Autodesk Inventor part; units mm, degrees
ref_plane "YZ Plane" through (0, 0, 0) normal (1, 0, 0) x (0, 1, 0)
ref_plane "XZ Plane" through (0, 0, 0) normal (0, 1, 0) x (-1, 0, 0)
ref_plane "XY Plane" through (0, 0, 0) normal (0, 0, 1) x (1, 0, 0)
sketch "Sketch1" plane through (0, 0, 0) normal (0, 1, 0) x (-1, 0, 0)
  line L0 (101.6, -101.6) -> (-101.6, -101.6)
  line L1 (-101.6, -101.6) -> (-101.6, 101.6)
  line L2 (-101.6, 101.6) -> (101.6, 101.6)
  line L3 (101.6, 101.6) -> (101.6, -101.6)
  line L4 (96.6, -96.6) -> (-96.6, -96.6)
  line L5 (-96.6, -96.6) -> (-96.6, 96.6)
  line L6 (-96.6, 96.6) -> (96.6, 96.6)
  line L7 (96.6, 96.6) -> (96.6, -96.6)
  line L8 (101.6, 101.6) -> (-40.4, 101.6)
  circle A0 centre (0, 0) radius 88.9
  circle A1 centre (0, 0) radius 109.3376
  line L9 (-40.4, 101.6) -> (-101.6, 40.4)
  line L10 (-45.4, 101.6) -> (-101.6, 45.4)
  line L11 (96.6, 96.6) -> (96.6, 101.6)
  line L12 (-45.4, 101.6) -> (-35.4, 101.6)
  line L13 (-35.4, 101.6) -> (-35.4, 96.6)
  line L14 (-35.4, 96.6) -> (-45.4, 96.6)
  line L15 (-45.4, 96.6) -> (-45.4, 101.6)
  circle A2 centre (0, 0) radius 111.3376
  point P0 (96.6, 51.2168)
  point P1 (101.6, 40.4)
  point P2 (101.6, -40.4)
  point P3 (96.6, -51.2168)
  point P4 (-96.6, 45.4)
  point P5 (-45.4, 96.6)
  dimension "d0" = 203.2
  dimension "d1" = 203.2
  dimension "d2" = 101.6
  dimension "d3" = 101.6
  dimension "d4" = 5
  dimension "d5" = 5
  dimension "d6" = 5
  dimension "d7" = 5
  dimension "d10" = 142
  dimension "d12" = 61.2
  dimension "d14" = 177.8
  dimension "d15" = 5
  dimension "d16" = 5
  dimension "d17" = 10
  dimension "d34" = 2
extrude "Extrusion1" add sketch "Sketch1" along normal blind 3 contours A2 L7 L4 | L4 A1 L7 A2 | L4 A1 L5 L9 L6 L7 | A2 L5 A1 L4 | L4 L5 A2 | A1 L6 A2 L7 | A2 L6 L7
sketch "Sketch5" plane through (0, 3, 0) normal (0, 1, 0) x (1, 0, 0)
  line L0 (-96.6, -96.6) -> (45.4, -96.6)
  circle A0 centre (0, 0) radius 88.9
  line L1 (96.6, -45.4) -> (96.6, 96.6)
  line L2 (96.6, 0) -> (89.1, 0)
  line L3 (89.1, 0) -> (89.1, 10)
  line L4 (89.1, 10) -> (96.6, 10)
  line L5 (96.6, 10) -> (96.6, 0)
  line L6 (89.1, 0) -> (96.6, 0)
  line L7 (96.6, 0) -> (96.6, -10)
  line L8 (96.6, -10) -> (89.1, -10)
  line L9 (89.1, -10) -> (89.1, 0)
  line L10 (0, 0) -> (96.6, 0)
  point P0 (10, -96.6)
  dimension "d52" = 7.5
  dimension "d53" = 7.5
  dimension "d54" = 10
  dimension "d55" = 10
extrude "Extrusion4" add sketch "Sketch5" along normal blind 15 contours L3 L4 L1 L2 | L2 L1 L8 L9
sketch "Sketch7" plane through (89.1, 3, 10) normal (0, 0, 1) x (1, 0, 0)
  line L0 (2, 10) -> (5.5, 10)
  line L1 (5.5, 10) -> (5.5, 3)
  line L2 (5.5, 3) -> (2, 3)
  line L3 (2, 3) -> (2, 10)
  line L4 (7.5, 0) -> (7.5, 15)
  line L5 (0, 0) -> (0, 15)
  line L6 (0, 15) -> (7.5, 15)
  point P0 (-89.1, -3)
  dimension "d56" = 3.5
  dimension "d57" = 2
  dimension "d58" = 2
  dimension "d59" = 5
  dimension "d60" = 7
extrude "Extrusion6" cut sketch "Sketch7" against normal through all
fillet "Fillet7" radius 3.175 2 edges at (96.6, 18, 0) (89.1, 18, 0)
sketch "Sketch8" plane through (0, 3, 0) normal (0, 1, 0) x (1, 0, 0)
  arc A0 (-101.6, -98.425) -> (-98.425, -101.6) centre (-98.425, -98.425) ccw
  line L0 (44.0849, 101.6) -> (-98.425, 101.6)
  line L1 (-101.6, 98.425) -> (-101.6, -98.425)
  line L2 (-101.6, -46.1) -> (-101.6, -76.6)
  line L3 (-96.6, -96.6) -> (-96.6, 96.6)
  line L4 (-96.6, -46.1) -> (-96.6, -76.6)
  line L5 (-101.6, -76.6) -> (-96.6, -76.6)
  line L6 (-101.6, -46.1) -> (-96.6, -46.1)
  line L7 (-98.425, -101.6) -> (101.6, -101.6)
  line L8 (0, 0) -> (-101.6, 0)
  line L9 (-101.6, 46.1) -> (-101.6, 76.6)
  line L10 (-96.6, 46.1) -> (-96.6, 76.6)
  line L11 (-101.6, 76.6) -> (-96.6, 76.6)
  line L12 (-101.6, 46.1) -> (-96.6, 46.1)
  line L13 (-96.6, -76.6) -> (-90.1, -76.6)
  line L14 (-90.1, -76.6) -> (-90.1, -46.1)
  line L15 (-90.1, -46.1) -> (-96.6, -46.1)
  line L16 (-96.6, -46.1) -> (-96.6, -76.6)
  arc A1 (-98.425, 101.6) -> (-101.6, 98.425) centre (-98.425, 98.425) ccw
  line L17 (-101.6, 46.1) -> (-101.6, 76.6)
  line L18 (-96.6, 46.1) -> (-96.6, 76.6)
  line L19 (-101.6, 76.6) -> (-96.6, 76.6)
  line L20 (-101.6, 46.1) -> (-96.6, 46.1)
  line L21 (-96.6, 76.6) -> (-90.1, 76.6)
  line L22 (-90.1, 76.6) -> (-90.1, 46.1)
  line L23 (-90.1, 46.1) -> (-96.6, 46.1)
  line L24 (-96.6, 46.1) -> (-96.6, 76.6)
  point P0 (-98.425, 98.425)
  point P1 (46.1, 101.6)
  point P2 (46.1, 96.6)
  point P3 (76.6, 96.6)
  point P4 (76.6, 101.6)
  point P5 (-46.1, 96.6)
  dimension "d64" = 30.5
  dimension "d65" = 25
  dimension "d66" = 6.5
extrude "Extrusion7" cut sketch "Sketch8" against normal through all contours L21 L22 L23 L3 | L15 L14 L13 L3
sketch "Sketch10" plane through (0, 0, 0) normal (0, -1, 0) x (1, 0, 0)
  line L0 (-90, -90) -> (-90, 90)
  line L1 (-90, 90) -> (90, 90)
  line L2 (90, 90) -> (90, -90)
  line L3 (90, -90) -> (-90, -90)
  circle A0 centre (-90, -90) radius 1
  circle A1 centre (-90, 90) radius 1
  circle A2 centre (90, -90) radius 1
  point P0 (0, 0)
  point P1 (0, 0)
  dimension "d76" = 90
  dimension "d77" = 90
  dimension "d78" = 90
  dimension "d79" = 90
  dimension "d80" = 2
  dimension "d81" = 2
  dimension "d82" = 2
hole "Hole1" at (90, 0, -90) at (-90, 0, 90) at (-90, 0, -90) direction (0, 1, 0) diameter 2.85 depth 4 tip angle 118 countersink diameter 5.2 countersink angle 90
equation "\"d1\" = d0"
properties part number "Box_Walls_2"
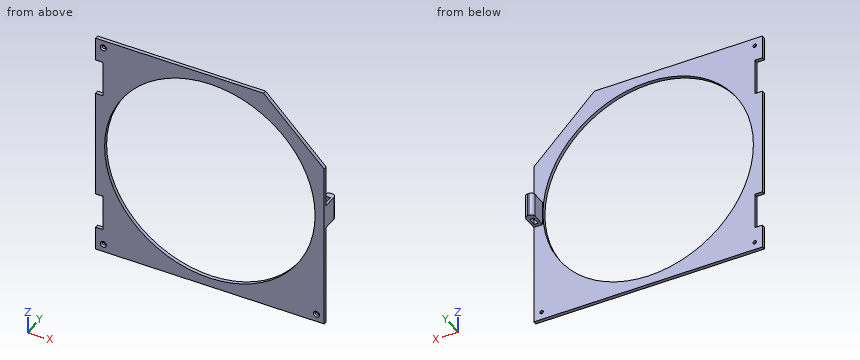
Part model, mm, in its own coordinate system. Coordinates: 2 decimals unless noted, no trailing zeros. Order: outer loops, then holes, each group sorted by start corner. A loop starts at its lowest first (then second) coordinate and runs counter-clockwise, first axis right, second up. Notation, with made-up numbers: (64.5, -19.75) - (71.5, -19.75) arc R28 cw to (71.5, 7.25) - close; hole circle Ø10 at (16.25, 8). An arc over 180 degrees is marked (long way). Return JSON: item names as keys, results as strings. Group by question number.
Item 1: Cut at B-B (z = 0). List the corners of the cut face in (x, y) (3 decimals).
Item 2: Pin check, flat tips, straight feed: pin 1 (1.7 mm diameter, centred on x = 90, z = -90, fed in from -Y); pin 2 (3.5 mm diameter, centred on x = -90, z = -90, fed in from -Y); pin 3 (6 mm diameter, centred on y = 9, z = 1.5, fed in from -X); pin 4 (3.5 mm diameter, centred on y = 1, z = 63, fed in from -X). Stop position of each tip, or through.
Item 3: Drill centre lines: probe 1 along X at (y, z) = (2.6, -90) (3 decimals); probe 2 along Z at (x, y) = (0, 2.15). Where is each one in solid material? Low to high. Write a range as from..to.
Item 4: Cut at A-A (y = 10). List the corners of the cut face in (x, z).
Item 5: Cut at C-C (x = 79). List the corners of the cut face in (y, z).
Check values:
{
 "1": {"outline": "(-96.6, 0) - (-88.9, 0) - (-88.9, 3) - (-96.6, 3) - close; (88.9, 0) - (96.6, 0) - (96.6, 14.825) arc R3.175 ccw to (93.425, 18) - (92.275, 18) arc R3.175 ccw to (89.1, 14.825) - (89.1, 3) - (88.9, 3) - close; hole (91.1, 6) - (94.6, 6) - (94.6, 13) - (91.1, 13) - close"},
 "2": {"pin 1": "passes through", "pin 2": "stops at y = 0.85", "pin 3": "stops at x = 89.1", "pin 4": "stops at x = -90.1"},
 "3": {"probe 1": "x = -96.6..-91.425, -88.575..88.575, 91.425..96.6", "probe 2": "z = -96.6..-88.9, 88.9..96.6"},
 "4": {"outline": "(89.1, -10) - (91.1, -10) - (91.1, 10) - (89.1, 10) - close; (94.6, -10) - (96.6, -10) - (96.6, 10) - (94.6, 10) - close"},
 "5": {"outline": "(0, -96.6) - (3, -96.6) - (3, -40.77) - (0, -40.77) - close; (0, 40.77) - (3, 40.77) - (3, 63) - (0, 63) - close"}
}
